Autodesk Inventor part; units mm, degrees
ref_plane "Work Plane1" through (0, 0, 2.75) normal (0, 0, 1) x (1, 0, 0)
ref_plane "YZ Plane" through (0, 0, 0) normal (1, 0, 0) x (0, 1, 0)
ref_plane "XZ Plane" through (0, 0, 0) normal (0, 1, 0) x (-1, 0, 0)
sketch "Sketch2" plane through (0, 0, 0) normal (0, 0, 1) x (1, 0, 0)
  line L0 (-4.2, 0) -> (4.2, 0) construction
  line L1 (0, -4.2) -> (0, 4.2) construction
  circle A0 centre (0, 0) radius 3
  line L2 (-3, 0) -> (3, 0)
  dimension "d0" = 6
revolve "Revolution1" add sketch "Sketch2" angle 360 about axis through (-10, 0, 0) along (1, 0, 0) picked at (0.7485, 0.6631) contours L2 A0
sketch "Sketch3" plane through (0, 0, 0) normal (0, 0, 1) x (1, 0, 0)
  circle A0 centre (0, 0) radius 1.5
  dimension "d2" = 3
extrude "Extrusion1" cut sketch "Sketch3" along normal through all both and the other way through all
ref_plane "Work Plane1" through (0, 0, 2.75) normal (0, 0, 1) x (1, 0, 0)
sketch "Sketch4" plane through (0, 0, 2.75) normal (0, 0, 1) x (1, 0, 0)
  circle A0 centre (0, 0) radius 1.5 construction
  circle A1 centre (0, 0) radius 1.5
  circle A2 centre (0, 0) radius 2.05
  dimension "d6" = 4.1
extrude "Extrusion2" add sketch "Sketch4" against normal up to surface
mirror "Mirror1" about plane through (0, 0, 0) normal (0, 0, 1) of "Extrusion2"
properties part number "Boule_tete_verin" material "Copper, Alloy"
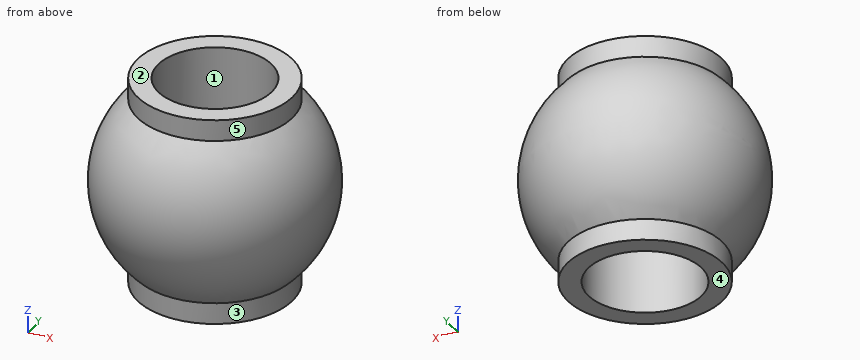
Geometry check sheet. Reference: the model listing, model coordinates, mm. Face numbers are marked on the shaded views. A direction names the side the tool comes from. Coordinates: 2 decimals unless noted, no trailing zeros. Order: outer loops, then holes, each group sorted by start corner. A loop starts at its lowest first (then second) coordinate and runs counter-clockwise, first axis right, second up.
Item 1: Tool access check on the marked faces 4 and 5. Record the directions out of +Z, -Z, +X, -X, +Y, -Y that give a thin tool (end or side, any length) a straight path to the whole face; none if there is none.
Item 2: Depth check by flat-ended pin: pin 1 (3 mm diameter, centred on x = 1, y = 0.5, fed in from -Z); pin 2 (3.5 mm diameter, centred on x = -0.5, y = 0.5, fed in from +Z); pin 3 (1 mm diameter, centred on y = 1, z = -2, fed in from +X). Enter the tip coordinate at first touch or a pass-through.
Item 3: Section check C-C (z = 1.4). Enter the section's corners in (x, y).
Item 4: Scan lines: line 1 along Y through (x, z) = (0, 0.05); line 2 along X through (y, z) = (-1.3, 1.7); line 3 along Y through (x, z) = (0, 2.3). Record each from-to range of solid material in increasing order.
Item 5: Mould release check, pull along X, two halves, no side actions. Record for the marked faces 1, 2 and 3: released by +X, released by -X, zero draft, split by the parting line, or undercut.
Item 6: Section check A-A (x = 0). Enter the section's corners in (y, z).
Item 7: Section check D-D (y = -1.75). Enter the section's corners in (x, z), plus the area to 3 significant figures.
Check sheet entries:
1. face 4: -Z, +X, -X, +Y, -Y
1. face 5: +Z
2. pin 1: stops at z = -2.75
2. pin 2: stops at z = 2.75
2. pin 3: stops at x = 2.45
3. outline: circle Ø5.31 at (0, 0); hole circle Ø3 at (0, 0)
4. line 1: y = -3 to -1.5, 1.5 to 3
4. line 2: x = -2.1 to -0.75, 0.75 to 2.1
4. line 3: y = -2.05 to -1.5, 1.5 to 2.05
5. face 1: undercut
5. face 2: zero draft
5. face 3: split by the parting line
6. outline: (-2.05, -2.75) - (-1.5, -2.75) - (-1.5, 2.75) - (-2.05, 2.75) - (-2.05, 2.19) arc R3 ccw to (-2.05, -2.19) - close; (1.5, -2.75) - (2.05, -2.75) - (2.05, -2.19) arc R3 ccw to (2.05, 2.19) - (2.05, 2.75) - (1.5, 2.75) - close
7. outline: (-1.07, -2.75) - (1.07, -2.75) - (1.07, -2.19) arc R2.44 ccw to (1.07, 2.19) - (1.07, 2.75) - (-1.07, 2.75) - (-1.07, 2.19) arc R2.44 ccw to (-1.07, -2.19) - close
7. area: 20.3 mm2
